Source: CAD feature listing. Evaluate the final solid. Frame: model axes, mm. Round coordinates to 2 decimals unless told otherwise and drop trailing zeros. Loops run counter-clockwise (first coordinate to the right, second up) from the corner with the lowest first, then second, coordinate; pieces in that order, holes last. Notation, with made-up numbers: (-25, 48) -> (-17, 48) arc R20 cw to (-17, 83) -> close; hole circle Ø9 at (43.25, 50.5). An arc over 180 degrees is marked (long way). Return JSON: item names as keys, results as strings. Group by question number.
Autodesk Inventor part; units mm, degrees
ref_plane "YZ Plane" through (0, 0, 0) normal (1, 0, 0) x (0, 1, 0)
ref_plane "XZ Plane" through (0, 0, 0) normal (0, 1, 0) x (-1, 0, 0)
ref_plane "XY Plane" through (0, 0, 0) normal (0, 0, 1) x (1, 0, 0)
sketch "Sketch1" plane through (0, 0, 0) normal (0, 0, 1) x (1, 0, 0)
  line L0 (-48.7274, 2.102) -> (2.0726, 2.102)
  line L1 (2.0726, 2.102) -> (2.0726, -1.073)
  line L2 (2.0726, -1.073) -> (-48.7274, -1.073)
  line L3 (-48.7274, -1.073) -> (-48.7274, 2.102)
  point P0 (0, 0)
  dimension "d0" = 3.175
  dimension "d1" = 50.8
extrude "Extrusion1" add sketch "Sketch1" along normal blind 136.5504
sketch "Sketch2" plane through (-48.7274, 2.102, 0) normal (0, 1, 0) x (1, 0, 0)
  circle A0 centre (12.7, -12.7) radius 1.7653
  circle A1 centre (38.1, -12.7) radius 1.7653
  circle A2 centre (12.7, -123.8504) radius 1.7653
  circle A3 centre (38.1, -123.8504) radius 1.7653
  line L0 (12.7, -123.8504) -> (38.1, -123.8504) construction
  line L1 (38.1, -123.8504) -> (38.1, -12.7) construction
  line L2 (38.1, -12.7) -> (12.7, -12.7) construction
  line L3 (12.7, -12.7) -> (12.7, -123.8504) construction
  line L4 (50.8, 0) -> (0, 0)
  line L5 (50.8, 0) -> (50.8, -136.5504)
  point P0 (48.7274, 0)
  dimension "d5" = 3.5306
  dimension "d6" = 111.1504
  dimension "d7" = 12.7
  dimension "d8" = 25.4
  dimension "d9" = 12.7
extrude "Extrusion2" cut sketch "Sketch2" against normal through all
sketch "Sketch3" plane through (-48.7274, 2.102, 0) normal (0, 1, 0) x (1, 0, 0)
  circle A0 centre (12.7, -79.4004) radius 1.7272
  circle A1 centre (38.1, -79.4004) radius 1.7272
  line L0 (12.7, -79.4004) -> (38.1, -79.4004) construction
  line L1 (0, 0) -> (0, -136.5504)
  circle A2 centre (12.7, -12.7) radius 1.7653
  circle A3 centre (12.7, -123.8504) radius 1.7653
  point P0 (48.7274, 0)
  point P1 (25.4, -79.4004)
  dimension "d12" = 3.4544
  dimension "d13" = 25.4
  dimension "d14" = 12.7
  dimension "d18" = 44.45
extrude "Extrusion3" cut sketch "Sketch3" against normal through all contours A0 | A1
equation "\"d3\" = d2"
equation "\"d2\" = 136.5504"
properties part number "Flat Bar KY"
(1) Mould query, pull axis Z, two halves, no side actions, for faces 1 (the face through (-48.727, 0, 67)), 2 (the face through (-24, 1, 136.55)), 3 (the face through (-36.26, 0.54, 122.1)). Classes: released by +Z, released by -Z, zero draft, split by the parting line, or undercut.
(2) Cut plane A-A (z = 12.7). Return loops of the section in (x, y).
(3) Ray query, line 1 (X direction, y = 0.9, z = 123.5); line 2 (Z direction, x = -11, y = -0.9); line 3 (Z direction, x = -9.5, y = 1.35). Return the intervals inside material, ascending.
(4) Pin query (flat end, axial travel): pin 1 (3 mm diameter, centred on x = -36.03, z = 79.4, fed in from -Y). Return the tip coordinate at first contact, or that it passes through.
Answers follow:
{
 "1": {"face 1": "zero draft", "face 2": "released by +Z", "face 3": "undercut"},
 "2": {"outline": "(-48.73, -1.07) -> (-37.79, -1.07) -> (-37.79, 2.1) -> (-48.73, 2.1) -> close; (-34.26, -1.07) -> (-12.39, -1.07) -> (-12.39, 2.1) -> (-34.26, 2.1) -> close; (-8.86, -1.07) -> (2.07, -1.07) -> (2.07, 2.1) -> (-8.86, 2.1) -> close"},
 "3": {"line 1": "-48.73 to -37.76, -34.3 to -12.36, -8.9 to 2.07", "line 2": "0 to 10.97, 14.43 to 77.71, 81.09 to 122.12, 125.58 to 136.55", "line 3": "0 to 11.34, 14.06 to 78.09, 80.71 to 122.49, 125.21 to 136.55"},
 "4": {"pin 1": "through"}
}
